```python
from build123d import *
from build123d.topology import SkipClean

# Parameters (mm, degrees)
BOSS_EXTRUDE1_DEPTH = 3
SKETCH3_R           = 4.1
CUT_EXTRUDE1_DEPTH  = 50
SKETCH1_3_R         = 6
BOSS_EXTRUDE2_DEPTH = 10
SKETCH1_4_R         = 6
BOSS_EXTRUDE3_DEPTH = 10
SKETCH1_5_R         = 6
BOSS_EXTRUDE8_DEPTH = 10
CHAMFER8_SIZE       = 5
CHAMFER8_SIZE_2     = 3.501037691
BOSS_EXTRUDE7_START = 1.9999999
BOSS_EXTRUDE7_DEPTH = 3.0000001


# Read off the part's stored shape, not the designer's step: Boss-Extrude7
with BuildPart() as part:
    # Sketch1 → Boss-Extrude1 (new body)
    with BuildSketch(Plane.XY):
        with BuildLine():
            ThreePointArc((-7.821268925, -1.68159222), (0.48240993, -7.985441795), (7.966824047, -0.727814955))
            Line((7.966824047, -0.727814955), (10.142674299, 23.089524856))
            ThreePointArc((10.142674299, 23.089524856), (9.947144202, 25.246709523), (8.998392886, 27.19389946))
            Line((8.998392886, 27.19389946), (-2.624147703, 42.972003574))
            ThreePointArc((-2.624147703, 42.972003574), (-5.470725652, 45.075885221), (-9.007898596, 45.209045145))
            Line((-9.007898596, 45.209045145), (-11.905676075, 44.432588009))
            ThreePointArc((-11.905676075, 44.432588009), (-15.472265696, 41.766039268), (-16.218713498, 37.375838886))
            Line((-16.218713498, 37.375838886), (-7.821268925, -1.68159222))
        make_face()
    extrude(amount=BOSS_EXTRUDE1_DEPTH)

    # Sketch3 → Cut-Extrude1 (cut)
    with BuildSketch(Plane.XY.offset(3)):
        Circle(SKETCH3_R)
    extrude(amount=-CUT_EXTRUDE1_DEPTH, mode=Mode.SUBTRACT)

    # Sketch1<3> → Boss-Extrude2 (add)
    with BuildSketch(Plane.XY):
        with Locations(Location((-10.352761804, 38.637033052, 0), (0, 0, 192.134016017))):
            Circle(SKETCH1_3_R)
    extrude(amount=BOSS_EXTRUDE2_DEPTH)

    # Sketch1<4> → Boss-Extrude3 (add)
    with BuildSketch(Plane.XY):
        with Locations((2.167556264, 25.701683368)):
            Circle(SKETCH1_4_R)
    extrude(amount=BOSS_EXTRUDE3_DEPTH)

    # Sketch1<5> → Boss-Extrude8 (add)
    with BuildSketch(Plane.XY):
        with Locations((2.25742631, 12.802500789)):
            Circle(SKETCH1_5_R)
    extrude(amount=BOSS_EXTRUDE8_DEPTH)

    # Sketch6 one side → Cut-Revolve1 (revolve, cut)
    with SkipClean():  # the faces are left unmerged after this step: merging them gives an invalid solid
        with BuildSketch(Plane(origin=(-10.352761804, 0, 0), x_dir=(0, 0, -1), z_dir=(1, 0, 0))):
            with BuildLine():
                ThreePointArc((-13, 34.637033052), (-10.171572875, 35.808605927), (-9, 38.637033052))
                ThreePointArc((-9, 38.637033052), (-10.171572875, 41.465460176), (-13, 42.637033052))
                Line((-13, 42.637033052), (-13, 34.637033052))
            make_face()
        revolve(axis=Axis((-10.352761804, 42.637033052, 13), (0, -1, 0)), mode=Mode.SUBTRACT)

    # Sketch7 one side → Cut-Revolve2 (revolve, cut)
    with SkipClean():  # the faces are left unmerged after this step: merging them gives an invalid solid
        with BuildSketch(Plane(origin=(2.167556264, 0, 0), x_dir=(0, 0, -1), z_dir=(1, 0, 0))):
            with BuildLine():
                ThreePointArc((-13, 21.701683368), (-10.171572875, 22.873256243), (-9, 25.701683368))
                ThreePointArc((-9, 25.701683368), (-10.171572875, 28.530110493), (-13, 29.701683368))
                Line((-13, 29.701683368), (-13, 21.701683368))
            make_face()
        revolve(axis=Axis((2.167556264, 29.701683368, 13), (0, -1, 0)), mode=Mode.SUBTRACT)

    # Sketch16 → Cut-Revolve3 (revolve, cut)
    with SkipClean():  # the faces are left unmerged after this step: merging them gives an invalid solid
        with BuildSketch(Plane(origin=(2.25742631, 0, 0), x_dir=(0, 0, -1), z_dir=(1, 0, 0))):
            with BuildLine():
                ThreePointArc((-9, 12.802500789), (-10.171572875, 15.630927914), (-13, 16.802500789))
                Line((-13, 16.802500789), (-13, 8.802500789))
                ThreePointArc((-13, 8.802500789), (-10.171572875, 9.974073664), (-9, 12.802500789))
            make_face()
            with BuildLine():
                Line((-13, 8.802500789), (-13, 16.802500789))
                ThreePointArc((-13, 16.802500789), (-17, 12.802500789), (-13, 8.802500789))
            make_face()
        revolve(axis=Axis((2.25742631, 16.802500789, 13), (0, -1, 0)), mode=Mode.SUBTRACT)

    # Chamfer8
    # the kernel refuses this chamfer: 5, 3.501037691 mm, written as the material it takes off along each edge
    with BuildSketch(Plane(origin=(-10.352761804, 38.637033052, 10), x_dir=(-0.9776586156884893, -0.21019902751931718, 0), z_dir=(-0.21019902751931718, 0.9776586156884893, 0))) as chamfer8_piece_1:
        Polygon((6, -CHAMFER8_SIZE), (6 - CHAMFER8_SIZE_2, 0), (6, 0), align=None)
    revolve(axis=Axis((-10.352761804, 38.637033052, 10), (0, 0, 1)), mode=Mode.SUBTRACT)
    with BuildSketch(Plane(origin=(2.167556264, 25.701683368, 10), x_dir=(1, 0, 0), z_dir=(0, -1, 0))) as chamfer8_piece_2:
        Polygon((6, -CHAMFER8_SIZE), (6 - CHAMFER8_SIZE_2, 0), (6, 0), align=None)
    revolve(axis=Axis((2.167556264, 25.701683368, 10), (0, 0, 1)), mode=Mode.SUBTRACT)
    with BuildSketch(Plane(origin=(2.25742631, 12.802500789, 10), x_dir=(1, 0, 0), z_dir=(0, -1, 0))) as chamfer8_piece_3:
        Polygon((6, -CHAMFER8_SIZE), (6 - CHAMFER8_SIZE_2, 0), (6, 0), align=None)
    revolve(axis=Axis((2.25742631, 12.802500789, 10), (0, 0, 1)), mode=Mode.SUBTRACT)

    # Boss-Extrude7 outline → Boss-Extrude7 (add)
    with BuildSketch(Plane.XY.offset(3).offset(BOSS_EXTRUDE7_START)):
        with BuildLine():
            ThreePointArc((-8.799847533, 32.841478094), (-4.557206846, 40.189947323), (-11.905676075, 44.43258801))
            Line((-11.905676075, 44.43258801), (-11.388037985, 42.500736357))
            ThreePointArc((-11.388037985, 42.500736357), (-6.489058499, 39.672309232), (-9.317485624, 34.773329746))
            Line((-9.317485624, 34.773329746), (-8.799847533, 32.841478094))
        make_face()
    extrude(amount=BOSS_EXTRUDE7_DEPTH)


solid = part.part
```
Part model, mm, in its own coordinate system. A direction names the side the tool comes from. Coordinates: 2 decimals unless noted, no trailing zeros. Order: outer loops, then holes, each group sorted by start corner. A loop starts at its lowest first (then second) coordinate and runs counter-clockwise, first axis right, second up. Notation, with made-up numbers: (62, 74.25) - (92, 74.25) arc R13 cw to (92, 86.25) - close; hole circle Ø8 at (81.5, 60). An arc over 180 degrees is marked (long way). Return JSON: item names as keys, results as strings. Group by question number.
Item 1: Which spindle directions (+Z, -Z, +X, -X, +Y, -Y) get a long thin tool onto all of the face, cutting with end or side? Do faces 1 (the face through (4.94, 20.38, 3.99)), 2 (the face through (-5.423, 45.059, 1.479)), 3 (the face through (-6, 40, 8)), 4 (the face through (-9.005, 33.606, 7.146)), 5 (the face through (-11.708, 43.695, 6.812)). Say none if no direction does.
Item 2: Drill centre lines: probe 1 along Z at (x, y) = (-9, 16); probe 2 along Y at (x, z) = (-1.75, 4.5); probe 3 along Y at (x, z) = (4.5, 6). Where is each one in solid material? Low to high. Write a range as from..to.
Item 3: Pull direction X, two halves, no side cores. Call faces 6 (the face through (-12.08, 18.12, 1.48)), 7 (the face through (-3, 19, 0)), 8 (the face through (-0.534, 4.065, 1.521)), 9 (the face through (9.04, 11.01, 1.48)): pulls with the +X half, pulls with the -X half, needs draft (parallel to the pull), parting line crosses it, or undercut.
Item 4: Cut at A-A (y = 0). List the corners of the cut face in (x, z).
Item 5: Cut at D-D (y = 6). List the corners of the cut face in (x, z).
Item 6: Cut at C-C (z = 6). List the corners of the cut face in (x, y).
Item 7: Cut at B-B (z = 3.75). List the corners of the cut face in (x, y).
Item 8: Pin check, flat tips, straight feed: pin 1 (5 mm diameter, centred on y = 14.5, z = 1, fed in from -X); pin 2 (6 mm diameter, centred on x = -1, y = -1, fed in from +Z); pin 3 (5 mm diameter, centred on x = -9.5, z = 1.5, fed in from -Y). Stop position of each tip, or through.
Check values:
{
 "1": {"face 1": "+Z", "face 2": "+Z, -Z, +Y", "face 3": "+Z, +X", "face 4": "+Z, -Y", "face 5": "+Z, -X"},
 "2": {"probe 1": "z = 0..3", "probe 2": "y = 8.34..17.27, 21.16..30.25", "probe 3": "y = 8..17.6, 20.94..30.46"},
 "3": {"face 6": "pulls with the -X half", "face 7": "needs draft", "face 8": "undercut", "face 9": "pulls with the +X half"},
 "4": {"outline": "(-8.18, 0) - (-4.1, 0) - (-4.1, 3) - (-8.18, 3) - close; (4.1, 0) - (8.03, 0) - (8.03, 3) - (4.1, 3) - close"},
 "5": {"outline": "(-9.47, 0) - (8.58, 0) - (8.58, 3) - (-9.47, 3) - close"},
 "6": {"outline": "(-11.91, 44.43) - (-11.72, 43.76) arc R5.3 ccw to (-8.98, 33.52) - (-8.8, 32.84) arc R6 ccw to start; circle Ø10.6 at (2.17, 25.7); circle Ø10.6 at (2.26, 12.8)"},
 "7": {"outline": "circle Ø12 at (-10.35, 38.64); circle Ø12 at (2.17, 25.7); circle Ø12 at (2.26, 12.8)"},
 "8": {"pin 1": "stops at x = -11.84", "pin 2": "stops at z = 3", "pin 3": "stops at y = -3.87"}
}
